Check sheet for the drawn part. Datum: minimum x, y, z corner. Units: mm. Round coordinates to 2 decimals unless told otherwise and drop trailing zeros. Write each loop counter-clockwise with the first axis right and the second up, starting at its lowest first coordinate (ties: lowest second). Pieces come first, ordered by that corner, then holes.
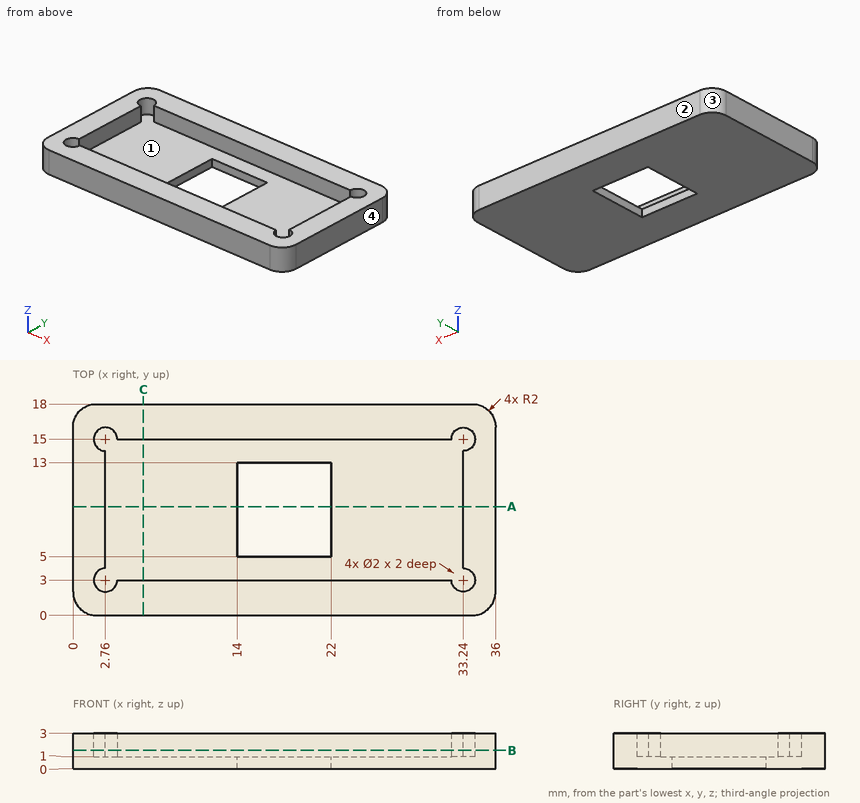
1. Sectioned sample at B-B, the plane z = 1.55. Enter the section's corners in (x, y).
2. Scan lines: line 1 along X through (y, z) = (9.75, 1.4); line 2 along X through (y, z) = (12, 0.85); line 3 along Y through (x, z) = (13, 1.5). Record each from-to range of solid material in increasing order.
3. Go/stop test with a flat-tipped pin: pin 1 (1.8 mm diameter, centred on x = 2.76, y = 15, fed in from +Z). Record where the tip stops, or that it passes through.
4. Sectioned sample at C-C, the plane x = 6. Enter the section's corners in (y, z), plus the area to 3 significant figures.
5. Release check for a two-part mould opening along X. For the marked faces 1, 2, 3 and 4 record: released by +X, released by -X, zero draft, split by the parting line, or undercut.
6. Sectioned sample at A-A, the plane y = 9.25. Enter the section's corners in (x, z).
Computed values:
1. outline: (0, 2) arc R2 ccw to (2, 0) - (34, 0) arc R2 ccw to (36, 2) - (36, 16) arc R2 ccw to (34, 18) - (2, 18) arc R2 ccw to (0, 16) - close; hole (2.76, 4) arc R1 ccw (long way) to (3.76, 3) - (32.24, 3) arc R1 ccw (long way) to (33.24, 4) - (33.24, 14) arc R1 ccw (long way) to (32.24, 15) - (3.76, 15) arc R1 ccw (long way) to (2.76, 14) - close
2. line 1: x = 0 to 2.76, 33.24 to 36
2. line 2: x = 0 to 14, 22 to 36
2. line 3: y = 0 to 3, 15 to 18
3. pin 1: stops at z = 1
4. outline: (0, 0) - (18, 0) - (18, 3) - (15, 3) - (15, 1) - (3, 1) - (3, 3) - (0, 3) - close
4. area: 30.0 mm2
5. face 1: undercut
5. face 2: zero draft
5. face 3: released by -X
5. face 4: released by +X
6. outline: (0, 0) - (14, 0) - (14, 1) - (2.76, 1) - (2.76, 3) - (0, 3) - close; (22, 0) - (36, 0) - (36, 3) - (33.24, 3) - (33.24, 1) - (22, 1) - close
